```python
from build123d import *

# Parameters (mm, degrees)
F0_R        = 5.75
F0_R_2      = 4.75
F1_DEPTH    = 4
F1_FACE_R   = 5.75
F1_FACE_R_2 = 4.75


with BuildPart() as f1:
    # F0 (on Top) → F1 (new body)
    with BuildSketch(Plane.XY):
        Circle(F0_R)
        Circle(F0_R_2, mode=Mode.SUBTRACT)
    extrude(amount=F1_DEPTH)

    # F5: sweep along a path in F4
    with BuildLine(Plane.XZ) as f5_path:
        Line((0, 4), (0, 12.7547773101))
        Line((0, 12.7547773101), (8, 12.7547773101))
    # F1_face (on face) → F5 (sweep)
    with BuildSketch(Plane.XY.offset(4)):
        Circle(F1_FACE_R)
        Circle(F1_FACE_R_2, mode=Mode.SUBTRACT)
    sweep(path=f5_path.line, transition=Transition.RIGHT)


solid = f1.part
```
Input: part model. Units: mm. Frame: model coordinates. Round coordinates to 2 decimals unless told otherwise and drop trailing zeros. Write each loop counter-clockwise with the first axis right and the second up, starting at its lowest first coordinate (ties: lowest second). Pieces come first, ordered by that corner, then holes. Notation, with made-up numbers: (23.5, 57.5) -> (38.5, 57.5) arc R24 ccw to (38.5, 84.5) -> close; hole circle Ø5 at (-17, 30). An arc over 180 degrees is marked (long way). Answer as CSV lines item,"result".
1. Section C-C (y = 3.25). Return the cut outline in (x, z).
Geometry says:
outline,"(-4.74, 0) -> (-3.46, 0) -> (-3.46, 16.22) -> (8, 16.22) -> (8, 17.5) -> (-4.74, 17.5) -> close; (3.46, 0) -> (4.74, 0) -> (4.74, 8.01) -> (8, 8.01) -> (8, 9.29) -> (3.46, 9.29) -> close"
2. Mould query, pull axis Y, two halves, no side actions, for faces 1 (the cylindrical face through (2.75, 0.25, 18.5)), 2 (the flat face through (8, -5, 14)), 3 (the cylindrical face through (3.1, 0.2, 17.5)). Classes: +Y half, -Y half, draft (parallel to the pull), parting line (faces both ways), or undercut.
Geometry says:
face 1,"parting line"
face 2,"draft"
face 3,"undercut"
3. Section A-A (y = 0). Return the cut outline in (x, z).
Geometry says:
outline,"(-5.75, 0) -> (-4.75, 0) -> (-4.75, 17.5) -> (8, 17.5) -> (8, 18.5) -> (-5.75, 18.5) -> close; (4.75, 0) -> (5.75, 0) -> (5.75, 7) -> (8, 7) -> (8, 8) -> (4.75, 8) -> close"
4. Contact query for flat-ended pins moving along their axis: P1, Ø2, axis at x = -3, y = 2.5, coming from the +Z side; P2, Ø4, axis at y = -2.5, z = 6.5, coming from the -X side; P3, Ø1, axis at x = 5, y = -4, coming from the +Z side. Output: stop coordinate, or through.
Geometry says:
P1,"stops at z = 18.31"
P2,"stops at x = -5.73"
P3,"stops at z = 17.32"
5. Ray query, L1, parallel to Y at x = -1.25, z = 5; L2, parallel to Y at x = 3.25, z = 5; L3, parallel to Z at x = 7, y = -3.25. Return the intervals inside material, ascending. Write a range as [from, to].
Geometry says:
L1,"y = [-5.61, -4.58], [4.58, 5.61]"
L2,"y = [-4.74, -3.46], [3.46, 4.74]"
L3,"z = [8.01, 9.29], [16.22, 17.5]"
6. Section D-D (x = 3). Return the cut outline in (y, z).
Geometry says:
outline,"(-4.91, 0) -> (-3.68, 0) -> (-3.68, 9.75) arc R4.75 cw (long way) to (3.68, 9.75) -> (3.68, 0) -> (4.91, 0) -> (4.91, 9.75) arc R5.75 ccw (long way) to (-4.91, 9.75) -> close"
7. Section B-B (z = 7.5). Return the cut outline in (x, y), plus the area to 3 significant figures.
Geometry says:
outline,"(5.25, -2.33) -> (8, -2.33) -> (8, 2.33) -> (5.25, 2.33) arc R5.75 ccw (long way) to start; hole circle Ø9.5 at (0, 0)"
area,"44.2 mm^2"
